Can you work these out from the model? Positions are in its coordinate system, mm. A direction names the side the tool comes from. Give positions to 0.01 mm unless a question says otherwise; leave off trailing zeros. Order: outer loops, then holes, each group sorted by start corner. A loop starts at its lowest first (then second) coordinate and runs counter-clockwise, first axis right, second up. Notation, with made-up numbers: (58, 60) - (92, 60) arc R27 cw to (92, 79) - close; hole circle Ø10 at (-4, -14). An arc over 180 degrees is marked (long way). Return JSON: item names as keys, results as strings.
```python
from build123d import *

# Parameters (mm, degrees)
SKETCH1_R           = 1.7
SKETCH1_R_2         = 2.5
BOSS_EXTRUDE1_DEPTH = 3
SKETCH1_11_R        = 4.15
CUT_EXTRUDE1_DEPTH  = 2
CUT_EXTRUDE2_START  = 0.5
CUT_EXTRUDE2_DEPTH  = 2.5


with BuildPart() as part:
    # Sketch1 → Boss-Extrude1 (new body)
    with BuildSketch(Plane(origin=(0, 0, 0), x_dir=(1, 0, 0), z_dir=(0, 1, 0))):
        with BuildLine():
            Line((12.840909091, 4.106221343), (3.681818182, 8.212442686))
            ThreePointArc((3.681818182, 8.212442686), (0, 9), (-3.681818182, 8.212442686))
            Line((-3.681818182, 8.212442686), (-12.840909091, 4.106221343))
            ThreePointArc((-12.840909091, 4.106221343), (-15.5, 0), (-12.840909091, -4.106221343))
            Line((-12.840909091, -4.106221343), (-3.681818182, -8.212442686))
            ThreePointArc((-3.681818182, -8.212442686), (0, -9), (3.681818182, -8.212442686))
            Line((3.681818182, -8.212442686), (12.840909091, -4.106221343))
            ThreePointArc((12.840909091, -4.106221343), (15.5, 0), (12.840909091, 4.106221343))
        make_face()
        with Locations(Location((-11, 0, 0), (0, 0, 270))):
            Circle(SKETCH1_R, mode=Mode.SUBTRACT)
        with Locations(Location((0, 0, 0), (0, 0, 270))):
            Circle(SKETCH1_R_2, mode=Mode.SUBTRACT)
        with Locations(Location((11, 0, 0), (0, 0, 270))):
            Circle(SKETCH1_R, mode=Mode.SUBTRACT)
    extrude(amount=BOSS_EXTRUDE1_DEPTH)

    # Sketch1<11> → Cut-Extrude1 (cut)
    with BuildSketch(Plane(origin=(0, 0, 0), x_dir=(1, 0, 0), z_dir=(0, 1, 0))):
        with Locations(Location((-11, 0, 0), (0, 0, 270))):
            Circle(SKETCH1_11_R)
        with Locations(Location((11, 0, 0), (0, 0, 270))):
            Circle(SKETCH1_11_R)
    extrude(amount=CUT_EXTRUDE1_DEPTH, mode=Mode.SUBTRACT)

    # Sketch1<12> → Cut-Extrude2 (cut)
    with BuildSketch(Plane(origin=(0, 0, 0), x_dir=(1, 0, 0), z_dir=(0, 1, 0)).offset(CUT_EXTRUDE2_START)):
        with BuildLine():
            Line((-5.25, 6.25), (-5.25, 0))
            Line((-5.25, 0), (-2.5, 0))
            ThreePointArc((-2.5, 0), (0, 2.5), (2.5, 0))
            Line((2.5, 0), (5.25, 0))
            Line((5.25, 0), (5.25, 6.25))
            Line((5.25, 6.25), (-5.25, 6.25))
        make_face()
        with BuildLine():
            Line((-2.5, 0), (-5.25, 0))
            Line((-5.25, 0), (-5.25, -6.25))
            Line((-5.25, -6.25), (5.25, -6.25))
            Line((5.25, -6.25), (5.25, 0))
            Line((5.25, 0), (2.5, 0))
            ThreePointArc((2.5, 0), (0, -2.5), (-2.5, 0))
        make_face()
    extrude(amount=CUT_EXTRUDE2_DEPTH, mode=Mode.SUBTRACT)


solid = part.part
```
1. For pin 1 Ø4.5 at (x, z) = (11, 0) entering from -Y; pin 2 Ø2.5 at (x, z) = (-11, 0) entering from -Y; pin 3 Ø1 at (x, y) = (-4, 1) entering from +Z; pin 4 Ø0.8 at (y, z) = (1, -2.5) entering from +X, each with a flat end and sliding along its axis, tell me the tip position at first contact or that it passes through.
Checks:
{"pin 1": "y = 2", "pin 2": "through", "pin 3": "z = 8.29", "pin 4": "x = 14.98"}
2. On a 3-axis mill with a long thin cutter (end or side, diameter ignored), from which of +Z, -Z, +X, -X, +Y, -Y can I reach the whole of each face in a straight line? I mean faces 4 (the face through (5.25, 2, 0)), 5 (the face through (0, 1, 9)), 6 (the face through (-13, 2, 0)). Say none if no direction works.
Checks:
{"face 4": "+Y", "face 5": "+Z, +Y, -Y", "face 6": "-Y"}
3. Thinking about a two-plate mould opening in Z: for faces 1 (the face through (-15.5, 1.5, -0.1)), 2 (the face through (-8.197, 1.479, -6.188)), 3 (the face through (9, 2, 0)), which applies, +Z half, -Z half, draft (parallel to the pull), parting line (faces both ways), or undercut?
Checks:
{"face 1": "parting line", "face 2": "-Z half", "face 3": "undercut"}
4. Suppose I cut it at D-D (z = 5.75). List the corners of the cut face in (x, y) for me, plus the area to 3 significant figures.
Checks:
{"outline": "(-9.17, 0) - (9.17, 0) - (9.17, 3) - (5.25, 3) - (5.25, 0.5) - (-5.25, 0.5) - (-5.25, 3) - (-9.17, 3) - close", "area": "28.8 mm^2"}
5. Suppose I cut it at C-C (y = 2.6). List the corners of the cut face in (x, z) for me.
Checks:
{"outline": "(-12.84, -4.11) - (-3.68, -8.21) arc R9 ccw to (3.68, -8.21) - (12.84, -4.11) arc R4.5 ccw to (12.84, 4.11) - (3.68, 8.21) arc R9 ccw to (-3.68, 8.21) - (-12.84, 4.11) arc R4.5 ccw to start; hole circle Ø3.4 at (-11, 0); hole (-5.25, -6.25) - (5.25, -6.25) - (5.25, 6.25) - (-5.25, 6.25) - close; hole circle Ø3.4 at (11, 0)"}
6. If I drill on L1, parallel to X at y = 0.45, z = 0; L2, parallel to X at y = 2.5, z = 0; L3, parallel to Y at x = 2, z = 5, over which ranges is the centre line in solid material (lowest first)? Write a range as [from, to].
Checks:
{"L1": "[-15.5, -15.15], [-6.85, -2.5], [2.5, 6.85], [15.15, 15.5]", "L2": "[-15.5, -12.7], [-9.3, -5.25], [5.25, 9.3], [12.7, 15.5]", "L3": "[0, 0.5]"}
7. Suppose I cut it at B-B (x = 0). List the corners of the cut face in (y, z) for me, plus the area to 4 significant figures.
Checks:
{"outline": "(0, -9) - (3, -9) - (3, -6.25) - (0.5, -6.25) - (0.5, -2.5) - (0, -2.5) - close; (0, 2.5) - (0.5, 2.5) - (0.5, 6.25) - (3, 6.25) - (3, 9) - (0, 9) - close", "area": "20.25 mm^2"}
8. Suppose I cut it at A-A (z = 0). List the corners of the cut face in (x, y) for me.
Checks:
{"outline": "(-15.5, 0) - (-15.15, 0) - (-15.15, 2) - (-12.7, 2) - (-12.7, 3) - (-15.5, 3) - close; (-9.3, 2) - (-6.85, 2) - (-6.85, 0) - (-2.5, 0) - (-2.5, 0.5) - (-5.25, 0.5) - (-5.25, 3) - (-9.3, 3) - close; (2.5, 0) - (6.85, 0) - (6.85, 2) - (9.3, 2) - (9.3, 3) - (5.25, 3) - (5.25, 0.5) - (2.5, 0.5) - close; (12.7, 2) - (15.15, 2) - (15.15, 0) - (15.5, 0) - (15.5, 3) - (12.7, 3) - close"}
